```python
from build123d import *

# Parameters (mm, degrees)
SKETCH1_R           = 0.7
SKETCH1_W           = 23
SKETCH1_H           = 12
BOSS_EXTRUDE1_DEPTH = 5


with BuildPart() as part:
    # Sketch1 → Boss-Extrude1 (new body)
    with BuildSketch(Plane(origin=(0, 0, 0), x_dir=(1, 0, 0), z_dir=(0, 1, 0))):
        Polygon((7.5, 10), (17.5, 10), (17.5, -10), (7.5, -10), (7.5, -15), (-7.5, -15), (-7.5, -10), (-17.5, -10), (-17.5, 10), (-7.5, 10), (-7.5, 15), (7.5, 15), align=None)
        with Locations(Location((-14, 0, 0), (0, 0, 270))):
            Circle(SKETCH1_R, mode=Mode.SUBTRACT)
        with Locations(Location((14, 0, 0), (0, 0, 270))):
            Circle(SKETCH1_R, mode=Mode.SUBTRACT)
        Rectangle(SKETCH1_W, SKETCH1_H, mode=Mode.SUBTRACT)
    extrude(amount=BOSS_EXTRUDE1_DEPTH)


solid = part.part
```
Could you check a few things on this model? Use its own coordinates, in mm. A direction names the side the tool comes from. Round coordinates to 2 decimals unless told otherwise and drop trailing zeros. Write each loop counter-clockwise with the first axis right and the second up, starting at its lowest first coordinate (ties: lowest second). Pieces come first, ordered by that corner, then holes.
(1) Suppose I cut it at D-D on z = 0. Write out the boundary of the cut face in (x, y), and give its area (3 significant figures).
Findings below:
outline: (-17.5, 0) - (-14.7, 0) - (-14.7, 5) - (-17.5, 5) - close; (-13.3, 0) - (-11.5, 0) - (-11.5, 5) - (-13.3, 5) - close; (11.5, 0) - (13.3, 0) - (13.3, 5) - (11.5, 5) - close; (14.7, 0) - (17.5, 0) - (17.5, 5) - (14.7, 5) - close
area: 46.0 mm2
(2) Thinking about a two-plate mould opening in X: for faces 6 (the face through (0, 2, 15)), 7 (the face through (0, 2, 6)), 8 (the face through (0, 2, -6)), 9 (the face through (17.5, 2, 0)), which applies, +X half, -X half, draft (parallel to the pull), parting line (faces both ways), or undercut?
Findings below:
face 6: draft
face 7: undercut
face 8: undercut
face 9: +X half
(3) If I drill on probe 1 along X at (y, z) = (1.5, 0); probe 2 along Z at (x, y) = (0.5, 2.35); probe 3 along Z at (x, y) = (-9.5, 0.6), over which ranges is the centre line in solid material (lowest first)?
Findings below:
probe 1: x = -17.5 to -14.7, -13.3 to -11.5, 11.5 to 13.3, 14.7 to 17.5
probe 2: z = -15 to -6, 6 to 15
probe 3: z = -10 to -6, 6 to 10
(4) Suppose I cut it at B-B on z = -3.75. Write out the boundary of the cut face in (x, y).
Findings below:
outline: (-17.5, 0) - (-11.5, 0) - (-11.5, 5) - (-17.5, 5) - close; (11.5, 0) - (17.5, 0) - (17.5, 5) - (11.5, 5) - close
(5) Suppose I cut it at C-C on y = 2.35. Write out the boundary of the cut face in (x, z), and give its area (3 significant figures).
Findings below:
outline: (-17.5, -10) - (-7.5, -10) - (-7.5, -15) - (7.5, -15) - (7.5, -10) - (17.5, -10) - (17.5, 10) - (7.5, 10) - (7.5, 15) - (-7.5, 15) - (-7.5, 10) - (-17.5, 10) - close; hole circle Ø1.4 at (-14, 0); hole (-11.5, -6) - (11.5, -6) - (11.5, 6) - (-11.5, 6) - close; hole circle Ø1.4 at (14, 0)
area: 571 mm2
(6) For pin 1 (1.5 mm diameter, centred on y = 2, z = -13, fed in from +X); pin 2 (2 mm diameter, centred on x = -9, y = 0.5, fed in from -Z); pin 3 (2.5 mm diameter, centred on y = 1.5, z = -12.5, fed in from -X); pin 4 (2 mm diameter, centred on x = 1, z = -3.5, fed in from -Y), each with a flat end and sliding along its axis, tell me the tip position at first contact or that it passes through.
Findings below:
pin 1: stops at x = 7.5
pin 2: stops at z = -10
pin 3: stops at x = -7.5
pin 4: passes through
(7) Suppose I cut it at A-A on x = -4. Write out the boundary of the cut face in (y, z).
Findings below:
outline: (0, -15) - (5, -15) - (5, -6) - (0, -6) - close; (0, 6) - (5, 6) - (5, 15) - (0, 15) - close
(8) Which directions (+Z, -Z, +X, -X, +Y, -Y) give clear straight access to the entire face, cutting with the end or side of a thin tool? Please do faces 1 (the face through (-12, 2, 10)), 2 (the face through (12, 2, -10)), 3 (the face through (11.5, 2, 0)), 4 (the face through (-13, 2, -10)), 5 (the face through (13, 2, 10)).
Findings below:
face 1: +Z, -X, +Y, -Y
face 2: -Z, +X, +Y, -Y
face 3: +Y, -Y
face 4: -Z, -X, +Y, -Y
face 5: +Z, +X, +Y, -Y
